from build123d import *

# Parameters (mm, degrees)
BOSS_EXTRUDE1_DEPTH   = 90
SKETCH4_R             = 1.5
SKETCH4_R_2           = 4
CUT_EXTRUDE1_DEPTH    = 31
SKETCH6_R             = 4
SKETCH6_R_2           = 1.5
CUT_EXTRUDE2_DEPTH    = 31
CROQUIS3_R            = 4
CROQUIS3_R_2          = 1.5
CORTAR_EXTRUIR1_DEPTH = 10
CROQUIS6_R            = 4
CROQUIS6_R_2          = 1.5
CORTAR_EXTRUIR2_DEPTH = 10


with BuildPart() as part:
    # Sketch3 → Boss-Extrude1 (new body)
    with BuildSketch(Plane.XY):
        with BuildLine():
            Line((-2, 0.049393959), (-41, 0.049393959))
            Line((-41, 0.049393959), (-41, 2.049393959))
            Line((-41, 2.049393959), (-2.618272552, 2.049393959))
            ThreePointArc((-2.618272552, 2.049393959), (-2.194008483, 2.22512989), (-2.018272552, 2.649393959))
            Line((-2.018272552, 2.649393959), (-2.018272552, 26.449393959))
            ThreePointArc((-2.018272552, 26.449393959), (-2.194008483, 26.873658027), (-2.618272552, 27.049393959))
            Line((-2.618272552, 27.049393959), (-41.018189082, 27.049393959))
            Line((-41.018189082, 27.049393959), (-41.018189082, 29.049393959))
            Line((-41.018189082, 29.049393959), (-2.018189082, 29.049393959))
            ThreePointArc((-2.018189082, 29.049393959), (-0.60397552, 28.463607521), (-0.018189082, 27.049393959))
            Line((-0.018189082, 27.049393959), (-0.018189082, 2.049393959))
            ThreePointArc((-0.018189082, 2.049393959), (-0.597554333, 0.64159652), (-2, 0.049393959))
        make_face()
    extrude(amount=BOSS_EXTRUDE1_DEPTH)

    # Sketch4 → Cut-Extrude1 (cut)
    with BuildSketch(Plane(origin=(0, 29.049393959, 0), x_dir=(1, 0, 0), z_dir=(0, 1, 0))):
        with Locations(Location((-29.018189082, -3, 0), (0, 0, 180))):
            Circle(SKETCH4_R)
        with Locations(Location((-36.018189082, -10, 0), (0, 0, 180))):
            Circle(SKETCH4_R)
        with Locations(Location((-29.018189082, -10, 0), (0, 0, 180))):
            Circle(SKETCH4_R_2)
        with Locations(Location((-22.018189082, -10, 0), (0, 0, 180))):
            Circle(SKETCH4_R)
        with Locations(Location((-29.018189082, -17, 0), (0, 0, 180))):
            Circle(SKETCH4_R)
    extrude(amount=-CUT_EXTRUDE1_DEPTH, mode=Mode.SUBTRACT)

    # Sketch6 → Cut-Extrude2 (cut)
    with BuildSketch(Plane(origin=(0, 29.049393959, 0), x_dir=(1, 0, 0), z_dir=(0, 1, 0))):
        with Locations(Location((-29.018189082, -45.498892055, 0), (0, 0, 180))):
            Circle(SKETCH6_R)
        with Locations(Location((-29.018189082, -80.498892055, 0), (0, 0, 180))):
            Circle(SKETCH6_R)
        with Locations(Location((-36.018189082, -45.498892055, 0), (0, 0, 180))):
            Circle(SKETCH6_R_2)
        with Locations(Location((-36.018189082, -80.498892055, 0), (0, 0, 180))):
            Circle(SKETCH6_R_2)
        with Locations((5.981810918, -52.498892055)):
            Circle(SKETCH6_R_2)
        with Locations(Location((-29.018189082, -52.498892055, 0), (0, 0, 180))):
            Circle(SKETCH6_R_2)
        with Locations((-22.018189082, -10.498892055)):
            Circle(SKETCH6_R_2)
        with Locations(Location((-22.018189082, -45.498892055, 0), (0, 0, 180))):
            Circle(SKETCH6_R_2)
        with Locations((-64.018189082, -38.498892055)):
            Circle(SKETCH6_R_2)
        with Locations(Location((-29.018189082, -38.498892055, 0), (0, 0, 180))):
            Circle(SKETCH6_R_2)
        with Locations(Location((-29.018189082, -73.498892055, 0), (0, 0, 180))):
            Circle(SKETCH6_R_2)
        with Locations(Location((-22.018189082, -80.498892055, 0), (0, 0, 180))):
            Circle(SKETCH6_R_2)
        with Locations(Location((-29.018189082, -87.498892055, 0), (0, 0, 180))):
            Circle(SKETCH6_R_2)
    extrude(amount=-CUT_EXTRUDE2_DEPTH, mode=Mode.SUBTRACT)

    # Croquis3 → Cortar-Extruir1 (cut)
    with BuildSketch(Plane(origin=(-0.018189082, 0, 0), x_dir=(0, 0, -1), z_dir=(1, 0, 0))):
        with Locations(Location((-45, 14.549393959, 0), (0, 0, 90))):
            Circle(CROQUIS3_R)
        with Locations(Location((-38, 14.549393959, 0), (0, 0, 90))):
            Circle(CROQUIS3_R_2)
        with Locations(Location((-45, 21.549393959, 0), (0, 0, 90))):
            Circle(CROQUIS3_R_2)
        with Locations(Location((-45, 7.549393959, 0), (0, 0, 90))):
            Circle(CROQUIS3_R_2)
        with Locations(Location((-52, 14.549393959, 0), (0, 0, 90))):
            Circle(CROQUIS3_R_2)
    extrude(amount=-CORTAR_EXTRUIR1_DEPTH, mode=Mode.SUBTRACT)

    # Croquis6 → Cortar-Extruir2 (cut)
    with BuildSketch(Plane(origin=(-0.018189082, 0, 0), x_dir=(0, 0, -1), z_dir=(1, 0, 0))):
        with Locations(Location((-10, 14.549393959, 0), (0, 0, 90))):
            Circle(CROQUIS6_R)
        with Locations(Location((-3, 14.549393959, 0), (0, 0, 90))):
            Circle(CROQUIS6_R_2)
        with Locations(Location((-17, 14.549393959, 0), (0, 0, 90))):
            Circle(CROQUIS6_R_2)
        with Locations(Location((-10, 21.549393959, 0), (0, 0, 90))):
            Circle(CROQUIS6_R_2)
        with Locations(Location((-10, 7.549393959, 0), (0, 0, 90))):
            Circle(CROQUIS6_R_2)
        with Locations((-87, 14.549393959)):
            Circle(CROQUIS6_R_2)
        with Locations((-80, 7.549393959)):
            Circle(CROQUIS6_R_2)
        with Locations((-80, 21.549393959)):
            Circle(CROQUIS6_R_2)
        with Locations((-80, 14.549393959)):
            Circle(CROQUIS6_R)
        with Locations((-73, 14.549393959)):
            Circle(CROQUIS6_R_2)
    extrude(amount=-CORTAR_EXTRUIR2_DEPTH, mode=Mode.SUBTRACT)


solid = part.part
The model under review builds one solid part; all positions refer to its coordinate system, in mm. A direction names the side the tool comes from. Round coordinates to 2 decimals unless told otherwise and drop trailing zeros. Write each loop counter-clockwise with the first axis right and the second up, starting at its lowest first coordinate (ties: lowest second). Pieces come first, ordered by that corner, then holes. Notation, with made-up numbers: M -13.5,27.25 L 34.5,27.25 A26 cw 34.5,50.25 Z; hole C -19,79.25 d3. An arc over 180 degrees is marked long. Answer as CSV lines item,"result". Start each with the question number.
Q1. Consider section B-B, the plane z = 35. Give the boundary of the cut face in (x, y).
Q2. Wall thickness on line 1 along Z through (x, y) = (-36, 1.75); line 2 along Y through (x, z) = (-12, 85); line 3 along X through (y, z) = (17, 60): over which ranges is each line inside the solid? List them lowest first.
Q3. Tool access review of faces 4 (the face through (-18, 2.049, 44)), 5 (the face through (-1, 15, 71.57)): name each direction out of +Z, -Z, +X, -X, +Y, -Y from which nothing blocks a thin tool from reaching the whole face with its end or side.
Q4. Clearance check with flat-ended pins moving along their axes: P1, Ø10.5, axis at x = -29.02, z = 10, coming from the -Y side; P2, Ø4, axis at y = 5.5, z = 31.5, coming from the -X side. State where each tip first meets the part, or that it passes through.
Q5. Consider section A-A, the plane z = 3. Give the boundary of the cut face in (x, y), then the cut area to 3 significant figures.
Q6. The part is to be moulded in two halves that separate along Z. For faces 1 (the face through (-27.52, 28.06, 17.07)), 2 (the face through (-1, 8.24, 43.67)), 3 (the face through (-0.018, 9, 44)), say which applies: +Z half, -Z half, draft (parallel to the pull), parting line (faces both ways), or undercut.
Q7. Consider section C-C, the plane x = -28.5. State how many separate pieces and enclosed holes the cut face has, then the cut area to 3 significant figures.
Result set:
1,outline,"M -41.02,27.05 L -2.62,27.05 A0.6 cw -2.02,26.45 L -2.02,2.65 A0.6 cw -2.62,2.05 L -41,2.05 L -41,0.05 L -2,0.05 A2 ccw -0.02,2.05 L -0.02,27.05 A2 ccw -2.02,29.05 L -41.02,29.05 Z"
2,line 1,"z = 0 to 8.5, 11.5 to 44, 47 to 79, 82 to 90"
2,line 2,"y = 0.05 to 2.05, 27.05 to 29.05"
2,line 3,"x = -2.02 to -0.02"
3,face 4,"+Z, -Z, -X"
3,face 5,"+X, -X"
4,P1,"stops at y = 0.05"
4,P2,"stops at x = -2.02"
5,outline,"M -41.02,27.05 L -30.52,27.05 L -30.52,29.05 L -41.02,29.05 Z; M -41,0.05 L -30.52,0.05 L -30.52,2.05 L -41,2.05 Z; M -27.52,0.05 L -2,0.05 A2 ccw -0.02,2.05 L -0.02,13.05 L -2.02,13.05 L -2.02,2.65 A0.6 cw -2.62,2.05 L -27.52,2.05 Z; M -27.52,27.05 L -2.62,27.05 A0.6 cw -2.02,26.45 L -2.02,16.05 L -0.02,16.05 L -0.02,27.05 A2 ccw -2.02,29.05 L -27.52,29.05 Z"
5,area,"194 mm²"
6,face 1,"undercut"
6,face 2,"undercut"
6,face 3,"draft"
7,separate pieces,"20"
7,enclosed holes,"0"
7,area,"197 mm²"
